Build history of the part. All positions in model axes, mm. Face numbers are marked on the shaded views. A direction names the side the tool comes from. Give positions to 0.01 mm unless a question says otherwise; leave off trailing zeros. Loops run counter-clockwise (first coordinate to the right, second up) from the corner with the lowest first, then second, coordinate; pieces in that order, holes last. Notation, with made-up numbers: (64.25, 32.25) -> (79.25, 32.25) arc R15 ccw to (79.25, 38.25) -> close; hole circle Ø11 at (26, 45.5). An arc over 180 degrees is marked (long way). Answer as a JSON object with one key per item and string values. Group by question number.
Q1. Drop flat-ended pins along their axis: pin 1 (5 mm diameter, centred on x = 92, z = 19, fed in from -Y); pin 2 (1 mm diameter, centred on x = 83, z = 24, fed in from +Y); pin 3 (2.5 mm diameter, centred on y = -15, z = 22, fed in from +X). Give the stop position or say it passes through.
Q2. Band-saw the part on D-D, the plane z = 21. Write the cut outline in (x, y).
Q3. Two-plate mould, pull along X, no slides. Class the marked faces 1, 2 and 3: pulls with the +X half, pulls with the -X half, needs draft (parallel to the pull), parting line crosses it, or undercut.
Q4. Band-saw the part on C-C, the plane x = 87.5. Write the cut outline in (y, z).
Q5. Tool access for the marked faces 4, 5 and 6: list every direction of +Z, -Z, +X, -X, +Y, -Y with a clear straight run to the whole face (end or side of a thin tool).
Q6. Wall check: probe 1 along X at (y, z) = (-16, 19.5); probe 2 along Y at (x, z) = (89, 26.25); probe 3 along Z at (x, y) = (96.75, -16.3). Give the ranges that are in metal, low to high. Write a range as from..to.
Q7. Band-saw the part on B-B, the plane z = 25.75. Write the cut outline in (x, y).
Q8. Band-saw the part on A-A, the plane y = -13.95. Write the cut outline in (x, z), plus the area to 3 significant figures.
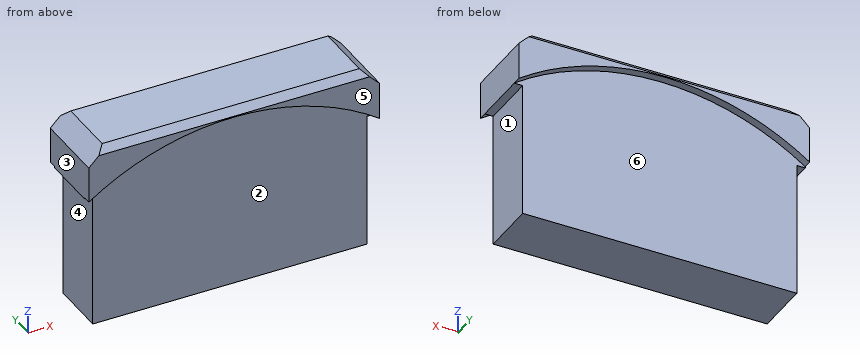
from build123d import *

# Parameters (mm, degrees)
SKETCH009_R         = 15
EXTRUDE003006_DEPTH = 0.5
SKETCH008_R         = 15
EXTRUDE003005_DEPTH = 0.5
BOX021_W            = 17.2
BOX021_H            = 4.3
BOX021_DEPTH        = 3.2
BOX020_W            = 16.2
BOX020_H            = 3.3
BOX020_DEPTH        = 8
CHAMFER002_SIZE     = 1
CHAMFER003_SIZE     = 0.4


with BuildPart() as extrude003006:
    # Sketch009 → Extrude003006 (new body)
    with BuildSketch(Plane.XZ):
        with Locations((89, 10.4)):
            Circle(SKETCH009_R)
    extrude(amount=EXTRUDE003006_DEPTH)


with BuildPart() as extrude003006_1:
    # Extrude003006 placement: moved
    add(extrude003006.part.moved(Location((0.05, -23.2, 0.15))))


with BuildPart() as extrude003005:
    # Sketch008 → Extrude003005 (new body)
    with BuildSketch(Plane.XZ):
        with Locations((89, 10.4)):
            Circle(SKETCH008_R)
    extrude(amount=EXTRUDE003005_DEPTH)


with BuildPart() as extrude003005_1:
    # Extrude003005 placement: moved
    add(extrude003005.part.moved(Location((0.05, -27, 0.15))))


with BuildPart() as tapa_puerta005:
    # Box021 → Box021 (new body)
    with BuildSketch(Plane(origin=(80.5, -27.5, 22.8), x_dir=(1, 0, 0), z_dir=(0, 0, 1))):
        with Locations((8.6, 2.15)):
            Rectangle(BOX021_W, BOX021_H)
    extrude(amount=BOX021_DEPTH)


with BuildPart() as tapa_pared:
    # Box020 → Box020 (new body)
    with BuildSketch(Plane(origin=(81, -27, 14.8), x_dir=(1, 0, 0), z_dir=(0, 0, 1))):
        with Locations((8.1, 1.65)):
            Rectangle(BOX020_W, BOX020_H)
    extrude(amount=BOX020_DEPTH)

    # Fusion009: union tapa_puerta005
    add(tapa_puerta005.part)

    # Cut005014017: cut Extrude003005
    add(extrude003005_1.part, mode=Mode.SUBTRACT)

    # Cut005014018: cut Extrude003006
    add(extrude003006_1.part, mode=Mode.SUBTRACT)

    # Chamfer002
    chamfer002_edges = [tapa_pared.edges().sort_by_distance(p)[0] for p in [
        (80.5, -25.35, 26),
        (97.7, -25.35, 26),
    ]]
    chamfer(chamfer002_edges, length=CHAMFER002_SIZE)

    # Chamfer003
    chamfer003_edges = [tapa_pared.edges().sort_by_distance(p)[0] for p in [
        (89.1, -27.5, 26),
        (89.1, -23.2, 26),
    ]]
    chamfer(chamfer003_edges, length=CHAMFER003_SIZE)


with BuildPart() as tapa_pared_1:
    # Chamfer003 placement: moved
    add(tapa_pared.part.moved(Location((0, 10.3, 2))))


solid = tapa_pared_1.part
Worked answers:
{
 "1": {"pin 1": "y = -16.7", "pin 2": "y = -13.4", "pin 3": "x = 97.2"},
 "2": {"outline": "(81, -16.7) -> (97.2, -16.7) -> (97.2, -13.4) -> (81, -13.4) -> close"},
 "3": {"face 1": "pulls with the +X half", "face 2": "undercut", "face 3": "pulls with the -X half"},
 "4": {"outline": "(-17.2, 27.47) -> (-16.7, 27.47) -> (-16.7, 16.8) -> (-13.4, 16.8) -> (-13.4, 27.47) -> (-12.9, 27.47) -> (-12.9, 27.6) -> (-13.3, 28) -> (-16.8, 28) -> (-17.2, 27.6) -> close"},
 "5": {"face 4": "-Z, -X, +Y, -Y", "face 5": "+Z, -Z, +X, -X, -Y", "face 6": "-Z, +Y"},
 "6": {"probe 1": "81..97.2", "probe 2": "-16.7..-13.4", "probe 3": "16.8..27.95"},
 "7": {"outline": "(80.5, -17.2) -> (81.93, -17.2) -> (81.93, -16.7) -> (96.17, -16.7) -> (96.17, -17.2) -> (97.7, -17.2) -> (97.7, -12.9) -> (96.17, -12.9) -> (96.17, -13.4) -> (81.93, -13.4) -> (81.93, -12.9) -> (80.5, -12.9) -> close"},
 "8": {"outline": "(80.5, 24.8) -> (81, 24.8) -> (81, 16.8) -> (97.2, 16.8) -> (97.2, 24.8) -> (97.7, 24.8) -> (97.7, 27) -> (96.7, 28) -> (81.5, 28) -> (80.5, 27) -> close", "area": "184 mm2"}
}
